Autodesk Inventor part; units mm, degrees
ref_plane "YZ Plane" through (0, 0, 0) normal (1, 0, 0) x (0, 1, 0)
ref_plane "XZ Plane" through (0, 0, 0) normal (0, 1, 0) x (-1, 0, 0)
ref_plane "XY Plane" through (0, 0, 0) normal (0, 0, 1) x (1, 0, 0)
sketch "Sketch1" plane through (0, 0, 0) normal (0, 1, 0) x (-1, 0, 0)
  line L0 (-9.525, 4.7625) -> (9.525, 4.7625)
  line L1 (9.525, 4.7625) -> (9.525, -4.7625)
  line L2 (9.525, -4.7625) -> (-9.525, -4.7625)
  line L3 (-9.525, -4.7625) -> (-9.525, 4.7625)
  line L4 (-9.525, 4.7625) -> (9.525, -4.7625) construction
  line L5 (9.525, 4.7625) -> (-9.525, -4.7625) construction
  point P0 (0, 0)
  dimension "d0" = 19.05
  dimension "d1" = 9.525
extrude "Plate1" add sketch "Sketch1" along normal blind 9.525
sketch "Sketch2" plane through (9.525, 0, -4.7625) normal (0, 0, -1) x (-1, 0, 0)
  line L0 (0, 0) -> (19.05, 0) construction
  line L1 (9.525, 0) -> (9.525, 9.525) construction
  line L2 (19.05, 9.525) -> (0, 9.525) construction
  point P0 (3.175, 6.35)
  point P1 (15.875, 6.35)
  dimension "d3" = 12.7
  dimension "d4" = 6.35
hole "Hole1" at (6.35, 6.35, -4.7625) at (-6.35, 6.35, -4.7625) direction (0, 0, 1) diameter 3.9624 end through all
sketch "Sketch3" plane through (0, 9.525, 0) normal (0, 1, 0) x (1, 0, 0)
  line L0 (-9.525, 4.7625) -> (9.525, 4.7625)
  point P0 (0, 0)
  point P1 (0, -1.5875)
  dimension "d19" = 6.35
hole "Hole2" at (0, 9.525, 1.5875) direction (0, -1, 0) diameter 3.9624 end through all
fillet "Corner Round1" radius 1.5875 4 edges at (-9.525, 4.7625, -4.7625) (-9.525, 4.7625, 4.7625) (9.525, 4.7625, -4.7625) (9.525, 4.7625, 4.7625)
equation "\"d10\" = Thickness"
equation "\"d2\" = Thickness"
equation "\"BendRadius\" = Thickness"
equation "\"BendReliefWidth\" = Thickness"
equation "\"BendReliefDepth\" = 0.5 * Thickness"
equation "\"CornerReliefSize\" = 4 * Thickness"
equation "\"MinimumRemnant\" = 2 * Thickness"
equation "\"TransitionRadius\" = BendRadius"
equation "\"JacobiRadiusSize\" = BendRadius"
equation "\"GapSize\" = Thickness"
properties part number "PLATE,NUTBLOCK,BACK" material "Aluminum 6061"
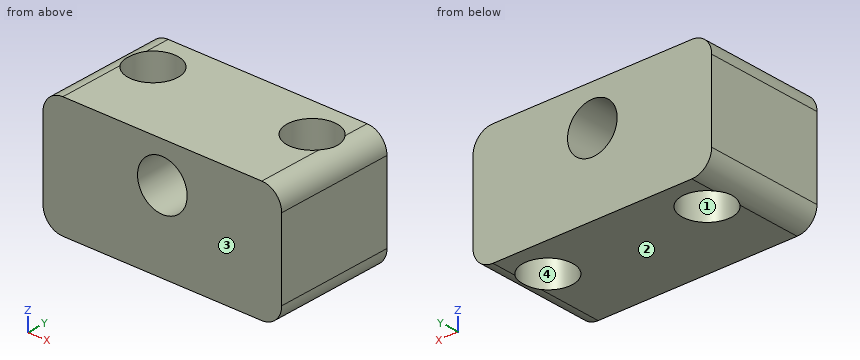
Input: part model. Units: mm. Frame: model coordinates. Face numbers are marked on the shaded views. Give positions to 0.01 mm unless a question says otherwise; leave off trailing zeros. Order: outer loops, then holes, each group sorted by start corner. A loop starts at its lowest first (then second) coordinate and runs counter-clockwise, first axis right, second up.
1. Cut plane C-C (y = 6.35). Return loops of the section in (x, z) (1 decimal), and give its area (3 significant figures).
Computed:
outline: (-9.5, -3.2) arc R1.6 ccw to (-8.3, -4.7) - (-8.3, 4.7) arc R1.6 ccw to (-9.5, 3.2) - close; (-4.4, -4.8) - (4.4, -4.8) - (4.4, 4.8) - (-4.4, 4.8) - close; (8.3, -4.7) arc R1.6 ccw to (9.5, -3.2) - (9.5, 3.2) arc R1.6 ccw to (8.3, 4.7) - close; hole circle Ø4 at (0, 1.6)
area: 91.5 mm2
2. Cut plane D-D (y = 8.75). Return loops of the section in (x, z) (1 decimal).
Computed:
outline: (-9.5, -3.2) arc R1.6 ccw to (-7.9, -4.8) - (7.9, -4.8) arc R1.6 ccw to (9.5, -3.2) - (9.5, 3.2) arc R1.6 ccw to (7.9, 4.8) - (-7.9, 4.8) arc R1.6 ccw to (-9.5, 3.2) - close; hole circle Ø4 at (0, 1.6)
3. Pin query (flat end, axial travel): pin 1 Ø3.5 at (x, z) = (0, 1.59) entering from +Y. Return the tip coordinate at first contact, or that it passes through.
Computed:
pin 1: passes through
4. Line query: probe 1 along X at (y, z) = (6.35, -2.5) (3 decimals); probe 2 along X at (y, z) = (6.35, 1.5) (3 decimals); probe 3 along Y at (x, z) = (-6.35, 1) (3 decimals). Output: solid intervals per line, ascending.
Computed:
probe 1: x = -9.525 to -8.331, -4.369 to 4.369, 8.331 to 9.525
probe 2: x = -9.525 to -8.331, -4.369 to -1.979, 1.979 to 4.369, 8.331 to 9.525
probe 3: y = 0 to 4.369, 8.331 to 9.525
5. Draft query along Y for the marked faces 1, 2, 3 and 4. Return one class per face: released by +Y, released by -Y, zero draft, split by the parting line, or undercut.
Computed:
face 1: undercut
face 2: zero draft
face 3: released by -Y
face 4: undercut
6. Cut plane B-B (z = 0). Return loops of the section in (x, y) (3 decimals), and give its area (3 significant figures).
Computed:
outline: (-9.525, 0) - (-1.185, 0) - (-1.185, 9.525) - (-9.525, 9.525) - close; (1.185, 0) - (9.525, 0) - (9.525, 9.525) - (1.185, 9.525) - close; hole circle Ø3.962 at (-6.35, 6.35); hole circle Ø3.962 at (6.35, 6.35)
area: 134 mm2
7. Cut plane A-A (x = -6.35). Return loops of the section in (y, z) (1 decimal).
Computed:
outline: (0, -4.8) - (4.4, -4.8) - (4.4, 4.8) - (0, 4.8) - close; (8.3, -4.8) - (9.5, -4.8) - (9.5, 4.8) - (8.3, 4.8) - close
